from build123d import *

# Parameters (mm, degrees)
SKETCH1_W           = 13.1
SKETCH1_H           = 4
BOSS_EXTRUDE1_DEPTH = 40
SKETCH2_W           = 21.1
SKETCH2_H           = 13
BOSS_EXTRUDE2_DEPTH = 4
SKETCH3_R           = 2
CUT_EXTRUDE1_DEPTH  = 50.571287052
SKETCH4_R           = 2
CUT_EXTRUDE2_DEPTH  = 60.306154824


with BuildPart() as part:
    # Sketch1 → Boss-Extrude1 (new body)
    with BuildSketch(Plane(origin=(0, 0, 0), x_dir=(1, 0, 0), z_dir=(0, 1, 0))):
        Polygon((-6.55, -15.1), (-6.55, -2), (-6.55, 2), (-10.55, 2), (-10.55, -15.1), align=None)
        Rectangle(SKETCH1_W, SKETCH1_H)
        Polygon((6.55, 2), (6.55, -2), (6.55, -15.1), (10.55, -15.1), (10.55, 2), align=None)
    extrude(amount=BOSS_EXTRUDE1_DEPTH)

    # Sketch2 → Boss-Extrude2 (add)
    with BuildSketch(Plane.XZ):
        Polygon((30.55, 15.1), (10.55, 15.1), (10.55, -2), (10.55, -15), (30.55, -15), align=None)
        with Locations((0, -8.5)):
            Rectangle(SKETCH2_W, SKETCH2_H)
        Polygon((-10.55, -15), (-10.55, -2), (-10.55, 15.1), (-30.55, 15.1), (-30.55, -15), align=None)
    extrude(amount=-BOSS_EXTRUDE2_DEPTH)

    # Sketch3 → Cut-Extrude1 (cut, through all)
    with BuildSketch(Plane(origin=(0, 4, 0), x_dir=(1, 0, 0), z_dir=(0, 1, 0))):
        with Locations(Location((-23.55, 8.5, 0), (0, 0, 270))):
            Circle(SKETCH3_R)
        with Locations(Location((23.55, 8.5, 0), (0, 0, 270))):
            Circle(SKETCH3_R)
    extrude(amount=-CUT_EXTRUDE1_DEPTH, mode=Mode.SUBTRACT)

    # Sketch4 → Cut-Extrude2 (cut, through all)
    with BuildSketch(Plane.ZY.offset(10.55)):
        with Locations((8.55, 9)):
            Circle(SKETCH4_R)
        with Locations((8.55, 32)):
            Circle(SKETCH4_R)
    extrude(amount=-CUT_EXTRUDE2_DEPTH, mode=Mode.SUBTRACT)


solid = part.part
Design review of the part built by this model. Coordinates are the model's own, in mm. A direction names the side the tool comes from. Give positions to 0.01 mm unless a question says otherwise; leave off trailing zeros. Write each loop counter-clockwise with the first axis right and the second up, starting at its lowest first coordinate (ties: lowest second). Pieces come first, ordered by that corner, then holes. Notation, with made-up numbers: M 62.5,85.25 L 88.5,85.25 A32 ccw 88.5,117.25 Z; hole C 31.5,70.25 d11. An arc over 180 degrees is marked long. Answer as a JSON object with one key per item and string values. Group by question number.
1) Clearance check with flat-ended pins moving along their axes: pin 1 Ø23 at (x, y) = (-0.5, 24.5) entering from -Z; pin 2 Ø3 at (y, z) = (9, 8.55) entering from -X; pin 3 Ø4.5 at (y, z) = (32, 8.55) entering from +X; pin 4 Ø10.5 at (x, y) = (-1, 19.5) entering from +Z. State where each tip first meets the part, or that it passes through.
2) We need section B-B (y = 3). Give the boundary of the cut face in (x, z).
3) We need section D-D (z = 13). Give the boundary of the cut face in (x, y).
4) Tool access review of faces 4 (the face through (-6.55, 20, 9)), 5 (the face through (10.55, 22, 7)), 6 (the face through (-10.55, 22, 6)), 7 (the face through (30.55, 2, 0)): name each direction out of +Z, -Z, +X, -X, +Y, -Y from which nothing blocks a thin tool from reaching the whole face with its end or side.
5) We need section A-A (z = -8.5). Give the boundary of the cut face in (x, y), and give its area (3 significant figures).
6) For line 1 along X through (y, z) = (1.8, -8.5); line 2 along Y through (x, z) = (-9.45, 8.55); line 3 along X through (y, z) = (32, 13), list the stretches that pass through material, from the lowest coordinate up.
7) Mouldability with a two-part tool opening along Z and no side actions: class faces 1 (the face through (6.55, 20, 8)), 2 (the face through (0, 20, 2)), 3 (the face through (-25.502, 2.028, -8.934)) as released by +Z, released by -Z, zero draft, split by the parting line, or undercut.
8) We need section C-C (x = -23.55). Give the boundary of the cut face in (y, z), and give its area (3 significant figures).
Answer key:
{
 "1": {"pin 1": "stops at z = -2", "pin 2": "passes through", "pin 3": "stops at x = 10.55", "pin 4": "stops at z = 2"},
 "2": {"outline": "M -30.55,-15 L 30.55,-15 L 30.55,15.1 L 6.55,15.1 L 6.55,2 L -6.55,2 L -6.55,15.1 L -30.55,15.1 Z; hole C -23.55,-8.5 d4; hole C 23.55,-8.5 d4"},
 "3": {"outline": "M -30.55,0 L -6.55,0 L -6.55,40 L -10.55,40 L -10.55,4 L -30.55,4 Z; M 6.55,0 L 30.55,0 L 30.55,4 L 10.55,4 L 10.55,40 L 6.55,40 Z"},
 "4": {"face 4": "+Z, +Y, -Y", "face 5": "+Z, -Z, +X, +Y", "face 6": "+Z, -Z, -X, +Y", "face 7": "+Z, -Z, +X, +Y, -Y"},
 "5": {"outline": "M -30.55,0 L -25.55,0 L -25.55,4 L -30.55,4 Z; M -21.55,0 L 21.55,0 L 21.55,4 L -21.55,4 Z; M 25.55,0 L 30.55,0 L 30.55,4 L 25.55,4 Z", "area": "212 mm²"},
 "6": {"line 1": "x = -30.55 to -25.55, -21.55 to 21.55, 25.55 to 30.55", "line 2": "y = 0 to 7, 11 to 30, 34 to 40", "line 3": "x = -10.55 to -6.55, 6.55 to 10.55"},
 "7": {"face 1": "zero draft", "face 2": "released by +Z", "face 3": "undercut"},
 "8": {"outline": "M 0,-15 L 4,-15 L 4,-10.5 L 0,-10.5 Z; M 0,-6.5 L 4,-6.5 L 4,15.1 L 0,15.1 Z", "area": "104 mm²"}
}
